Work out the finished part from the listing and answer in its coordinate system (mm). Coordinates: 2 decimals unless noted, no trailing zeros. Order: outer loops, then holes, each group sorted by start corner. A loop starts at its lowest first (then second) coordinate and runs counter-clockwise, first axis right, second up.
Autodesk Fusion 360 part; units mm, degrees
sketch "Sketch1" plane through (0, 0, 0) normal (0, 0, 1) x (1, 0, 0)
  line L0 (-85.1, 55.6) -> (85.1, 55.6)
  line L1 (85.1, 55.6) -> (85.1, -55.6)
  line L2 (85.1, -55.6) -> (-85.1, -55.6)
  line L3 (-85.1, -55.6) -> (-85.1, 55.6)
  line L4 (-85.1, 55.6) -> (85.1, -55.6) construction
  line L5 (85.1, 55.6) -> (-85.1, -55.6) construction
  line L6 (-84.0199, 54.3533) -> (83.7801, 54.3533)
  line L7 (83.7801, 54.3533) -> (83.7801, -52.7367)
  line L8 (83.7801, -52.7367) -> (-84.0199, -52.7367)
  line L9 (-84.0199, -52.7367) -> (-84.0199, 54.3533)
  line L10 (-83.0921, 52.8533) -> (81.7079, 52.8533)
  line L11 (81.7079, 52.8533) -> (81.7079, -51.2367)
  line L12 (81.7079, -51.2367) -> (-83.0921, -51.2367)
  line L13 (-83.0921, -51.2367) -> (-83.0921, 52.8533)
  line L14 (-82.6768, 52.0533) -> (80.5232, 52.0533)
  line L15 (80.5232, 52.0533) -> (80.5232, -45.8667)
  line L16 (-82.6768, 52.0533) -> (-82.6768, -45.8667)
  line L17 (-82.6768, -45.8667) -> (80.5232, -45.8667)
  dimension "d1" = 170.2
  dimension "d2" = 111.2
  dimension "d5" = 107.09
  dimension "d9" = 164.8
  dimension "d10" = 104.09
  dimension "d12" = 163.2
  dimension "d14" = 97.92
extrude "Extrude1" add sketch "Sketch1" along normal blind 0.7 contours L0 L1 L2 L3
extrude "Extrude2" add sketch "Sketch1" along normal blind 0.13 contours L6 L7 L8 L9
extrude "Extrude3" add sketch "Sketch1" along normal blind 0.07 contours L10 L11 L12 L13
extrude "Extrude4" add sketch "Sketch1" along normal blind 1.18 contours L14 L15 L16 L17
1. Consider probe 1 along X at (y, z) = (42, 0.35); probe 2 along Y at (x, z) = (-71.5, 0.2); probe 3 along Y at (x, z) = (-29.5, 0.9). Determine where each line is inside the solid, lowest interval first.
2. The part is cut by section B-B (x = -55). Determine the outline of the cut face in (y, z).
3. The part is cut by section C-C (y = 29.5). Determine the outline of the cut face in (x, z), plus the area to 3 significant figures.
4. The part is cut by section A-A (z = 0.45). Determine the outline of the cut face in (x, y), plus the area to 3 significant figures.
5. A flat-ended cylindrical pin translates along its axis: pin 1 (5 mm diameter, centred on x = 24.5, y = 17, fed in from -Z). Find the tip coordinate at first contact, or state that the pin passes through.
Worked out:
1. probe 1: x = -85.1 to -84.02, -82.68 to 80.52, 83.78 to 85.1
1. probe 2: y = -55.6 to -52.74, -45.87 to 52.05, 54.35 to 55.6
1. probe 3: y = -45.87 to 52.05
2. outline: (-55.6, 0) - (55.6, 0) - (55.6, 0.7) - (54.35, 0.7) - (54.35, 0.13) - (52.85, 0.13) - (52.85, 0.07) - (52.05, 0.07) - (52.05, 1.18) - (-45.87, 1.18) - (-45.87, 0.07) - (-51.24, 0.07) - (-51.24, 0.13) - (-52.74, 0.13) - (-52.74, 0.7) - (-55.6, 0.7) - close
3. outline: (-85.1, 0) - (85.1, 0) - (85.1, 0.7) - (83.78, 0.7) - (83.78, 0.13) - (81.71, 0.13) - (81.71, 0.07) - (80.52, 0.07) - (80.52, 1.18) - (-82.68, 1.18) - (-82.68, 0.07) - (-83.09, 0.07) - (-83.09, 0.13) - (-84.02, 0.13) - (-84.02, 0.7) - (-85.1, 0.7) - close
3. area: 195 mm2
4. outline: (-85.1, -55.6) - (85.1, -55.6) - (85.1, 55.6) - (-85.1, 55.6) - close; (-82.68, -45.87) - (80.52, -45.87) - (80.52, 52.05) - (-82.68, 52.05) - close; hole (-84.02, -52.74) - (83.78, -52.74) - (83.78, 54.35) - (-84.02, 54.35) - close
4. area: 16,900 mm2
5. pin 1: stops at z = 0
